from build123d import *

# Parameters (mm, degrees)
F0_R     = 38.1
F1_DEPTH = 22.225
F2_R     = 6.35
F3_DEPTH = 35.49923
F4_R     = 12.7
F4_R_2   = 6.35
F5_DEPTH = 22.225


with BuildPart() as f1:
    # F0 (on Top) → F1 (new body)
    with BuildSketch(Plane.XY):
        Circle(F0_R)
    extrude(amount=F1_DEPTH)

    # F2 (on face) → F3 (cut)
    with BuildSketch(Plane.XY.offset(22.225)):
        Circle(F2_R)
    extrude(amount=-F3_DEPTH, mode=Mode.SUBTRACT)

    # F4 (on face) → F5 (join)
    with BuildSketch(Plane(origin=(0, 0, 0), x_dir=(1, 0, 0), z_dir=(0, 0, -1))):
        Circle(F4_R)
        Circle(F4_R_2, mode=Mode.SUBTRACT)
    extrude(amount=F5_DEPTH)


solid = f1.part
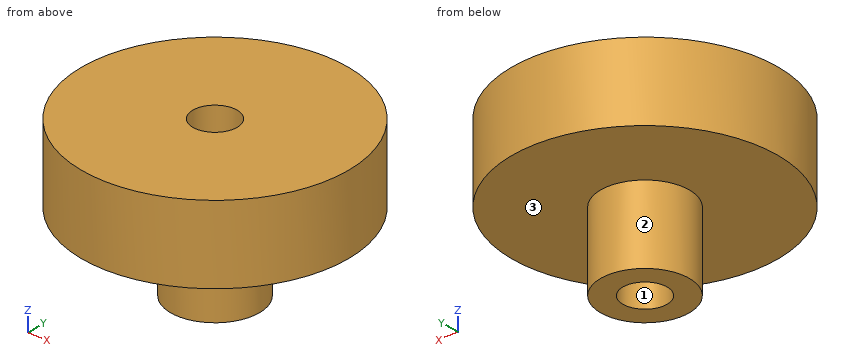
The listing builds one solid part. Answer for the finished solid, in the listing's coordinates (mm). Face numbers are marked on the shaded views. Round coordinates to 2 decimals unless told otherwise and drop trailing zeros. Order: outer loops, then holes, each group sorted by start corner. A loop starts at its lowest first (then second) coordinate and runs counter-clockwise, first axis right, second up. Notation, with made-up numbers: (-1, -27.5) - (11, -27.5) arc R20 cw to (11, -18.5) - close; hole circle Ø6 at (73, 13.5). An arc over 180 degrees is marked (long way). Write item = value, one per line. Start each with the question number.
1) For a pull along Y with two mould halves and no side action, classify the marked faces 1, 2 and 3 as released by +Y, released by -Y, zero draft, split by the parting line, or undercut.
2) Straight lines are drawn through the part: L1, parallel to Y at x = 0, z = -10; L2, parallel to Y at x = 0, z = 12.5; L3, parallel to Z at x = 3.5, y = 27 (3 decimals). For each, find the intervals that lie inside material, in ascending order.
3) Given pin 1 (4 mm diameter, centred on y = -22, z = 11.5, fed in from +X); pin 2 (1.5 mm diameter, centred on x = 16.5, y = 24.5, fed in from -Z); pin 3 (3 mm diameter, centred on x = 30.5, z = 15.5, fed in from +Y); pin 4 (10 mm diameter, centred on x = 0, y = 0, fed in from -Z), each flat-ended and moving along its own axis, determine where each tip first touches the part or whether it passes through.
4) Section A-A, the plane x = 0 is taken. Write down the section's boundary in (y, z) (3 decimals), plus the area to 3 significant figures.
5) Section C-C, the plane z = 15.5 is taken. Write down the section's boundary in (x, y).
6) Section D-D, the plane x = 10.5 is taken. Write down the section's boundary in (y, z) (3 decimals), plus the area to 3 significant figures.
Results list:
q1.face_1 = undercut
q1.face_2 = split by the parting line
q1.face_3 = zero draft
q2.L1 = -12.7 to -6.35, 6.35 to 12.7
q2.L2 = -38.1 to -6.35, 6.35 to 38.1
q2.L3 = 0 to 22.225
q3.pin_1 = 32.43
q3.pin_2 = 0
q3.pin_3 = 24.71
q3.pin_4 = through
q4.outline = (-38.1, 0) - (-12.7, 0) - (-12.7, -22.225) - (-6.35, -22.225) - (-6.35, 22.225) - (-38.1, 22.225) - close; (6.35, -22.225) - (12.7, -22.225) - (12.7, 0) - (38.1, 0) - (38.1, 22.225) - (6.35, 22.225) - close
q4.area = 1,690 mm^2
q5.outline = circle Ø76.2 at (0, 0); hole circle Ø12.7 at (0, 0)
q6.outline = (-36.625, 0) - (-7.144, 0) - (-7.144, -22.225) - (7.144, -22.225) - (7.144, 0) - (36.625, 0) - (36.625, 22.225) - (-36.625, 22.225) - close
q6.area = 1,950 mm^2
